Could you check a few things on this model? Use its own coordinates, in mm. A direction names the side the tool comes from. Round coordinates to 2 decimals unless told otherwise and drop trailing zeros. Loops run counter-clockwise (first coordinate to the right, second up) from the corner with the lowest first, then second, coordinate; pieces in that order, holes last. Notation, with made-up numbers: M 81.5,-32 L 126.5,-32 A24 cw 126.5,-8 Z; hole C -18,35 d1. An arc over 180 degrees is marked long. Answer in a Markdown table with one row per item.
```python
from build123d import *

# Parameters (mm, degrees)
SKETCH2_W           = 25
SKETCH2_H           = 35
BOSS_EXTRUDE2_DEPTH = 35
SKETCH3_W           = 25
SKETCH3_H           = 25
CUT_EXTRUDE1_DEPTH  = 25
SKETCH5_W           = 25
SKETCH5_H           = 10
CUT_EXTRUDE2_DEPTH  = 15
SKETCH6_R           = 1
CUT_EXTRUDE3_DEPTH  = 15
SKETCH7_W           = 25
SKETCH7_H           = 20
CUT_EXTRUDE4_DEPTH  = 7
SKETCH9_R           = 1
CUT_EXTRUDE6_DEPTH  = 15
SKETCH10_W          = 25
SKETCH10_H          = 28
CUT_EXTRUDE7_DEPTH  = 5


with BuildPart() as part:
    # Sketch2 → Boss-Extrude2 (new body)
    with BuildSketch(Plane.XY):
        with Locations((-5.377094972, 0.097765363)):
            Rectangle(SKETCH2_W, SKETCH2_H)
    extrude(amount=BOSS_EXTRUDE2_DEPTH)

    # Sketch3 → Cut-Extrude1 (cut)
    with BuildSketch(Plane.XY.offset(35)):
        with Locations((-5.377094972, 5.097765363)):
            Rectangle(SKETCH3_W, SKETCH3_H)
    extrude(amount=-CUT_EXTRUDE1_DEPTH, mode=Mode.SUBTRACT)

    # Sketch5 → Cut-Extrude2 (cut)
    with BuildSketch(Plane.XY.offset(35)):
        with Locations((-5.377094972, -12.402234637)):
            Rectangle(SKETCH5_W, SKETCH5_H)
    extrude(amount=-CUT_EXTRUDE2_DEPTH, mode=Mode.SUBTRACT)

    # Sketch6 → Cut-Extrude3 (cut)
    with BuildSketch(Plane(origin=(0, -7.402234637, 0), x_dir=(1, 0, 0), z_dir=(0, 1, 0))):
        with Locations((-14.877924678, -15)):
            Circle(SKETCH6_R)
        with Locations((4.122905028, -15)):
            Circle(SKETCH6_R)
    extrude(amount=-CUT_EXTRUDE3_DEPTH, mode=Mode.SUBTRACT)

    # Sketch7 → Cut-Extrude4 (cut)
    with BuildSketch(Plane.XZ.offset(17.402234637)):
        with Locations((-5.377094972, 10)):
            Rectangle(SKETCH7_W, SKETCH7_H)
    extrude(amount=-CUT_EXTRUDE4_DEPTH, mode=Mode.SUBTRACT)

    # Sketch9 → Cut-Extrude6 (cut)
    with BuildSketch(Plane.XY.offset(10)):
        with Locations((-15.877094972, 15.597765363)):
            Circle(SKETCH9_R)
        with Locations((5.122905028, 15.597765363)):
            Circle(SKETCH9_R)
        with Locations((-15.877094972, 3.597765363)):
            Circle(SKETCH9_R)
        with Locations((5.122905028, 3.597765363)):
            Circle(SKETCH9_R)
    extrude(amount=-CUT_EXTRUDE6_DEPTH, mode=Mode.SUBTRACT)

    # Sketch10 → Cut-Extrude7 (cut)
    with BuildSketch(Plane(origin=(0, 0, 0), x_dir=(-1, 0, 0), z_dir=(0, 0, -1))):
        with Locations((5.377094972, 3.597765363)):
            Rectangle(SKETCH10_W, SKETCH10_H)
    extrude(amount=-CUT_EXTRUDE7_DEPTH, mode=Mode.SUBTRACT)


solid = part.part
```
1) Will these pins go through, and if not, where does the flat tip stop? P1, Ø1.2, axis at x = 5.12, y = 15.6, coming from the +Z side; P2, Ø3, axis at x = -4, z = 13, coming from the +Y side; P3, Ø6, axis at x = -2, y = 14, coming from the +Z side; P4, Ø8, axis at y = -3.5, z = 12.5, coming from the -X side.
Computed:
| item | result |
|---|---|
| P1 | passes through |
| P2 | stops at y = -7.4 |
| P3 | stops at z = 10 |
| P4 | stops at x = -17.88 |
2) If we mould it in two halves opening along X, with no side actions, what happens to faces 3 (the face through (4.91, 14.62, 7.54)), 4 (the face through (-17.877, 0, 9)), 5 (the face through (-5, 4, 5))? For each: released by +X, released by -X, zero draft, split by the parting line, or undercut.
Computed:
| item | result |
|---|---|
| face 3 | undercut |
| face 4 | released by -X |
| face 5 | zero draft |
3) I want a section at A-A, the plane z = 15. Please give me the cut outline in (x, y), plus the area to 3 significant figures.
Computed:
| item | result |
|---|---|
| outline | M -17.88,-10.4 L -15.88,-10.4 L -15.88,-7.4 L -17.88,-7.4 Z; M -13.88,-10.4 L 3.12,-10.4 L 3.12,-7.4 L -13.88,-7.4 Z; M 5.12,-10.4 L 7.12,-10.4 L 7.12,-7.4 L 5.12,-7.4 Z |
| area | 63.0 mm² |
4) I want a section at C-C, the plane y = 15. Please give me the cut outline in (x, z), plus the area to 3 significant figures.
Computed:
| item | result |
|---|---|
| outline | M -17.88,5 L -16.68,5 L -16.68,10 L -17.88,10 Z; M -15.08,5 L 4.32,5 L 4.32,10 L -15.08,10 Z; M 5.92,5 L 7.12,5 L 7.12,10 L 5.92,10 Z |
| area | 109 mm² |
5) I want a section at D-D, the plane x = -9.75. Please give me the cut outline in (y, z).
Computed:
| item | result |
|---|---|
| outline | M -10.4,5 L 17.6,5 L 17.6,10 L -7.4,10 L -7.4,20 L -10.4,20 Z |
6) I want a section at B-B, the plane x = -14.5. Please give me the cut outline in (y, z).
Computed:
| item | result |
|---|---|
| outline | M -10.4,5 L 17.6,5 L 17.6,10 L -7.4,10 L -7.4,14.07 L -10.4,14.07 Z; M -10.4,15.93 L -7.4,15.93 L -7.4,20 L -10.4,20 Z |
7) I need wall thicknesses on line 1 (X direction, y = -9.55, z = 15); line 2 (Y direction, x = -15.5, z = 7.5); line 3 (Y direction, x = -16.75, z = 16.5). Which ranges of each line are inside material? Lowest first, please.
Computed:
| item | result |
|---|---|
| line 1 | x = -17.88 to -15.88, -13.88 to 3.12, 5.12 to 7.12 |
| line 2 | y = -10.4 to 2.67, 4.52 to 14.67, 16.52 to 17.6 |
| line 3 | y = -10.4 to -7.4 |
8) Which directions (+Z, -Z, +X, -X, +Y, -Y) give clear straight access to the entire face, cutting with the end or side of a thin tool? Please do faces 1 (the face through (6.077, 3.898, 7.535)), 2 (the face through (-6, 5, 10)).
Computed:
| item | result |
|---|---|
| face 1 | +Z, -Z |
| face 2 | +Z, +X, -X, +Y |
